The listing builds one solid part. Answer for the finished solid, in the listing's coordinates (mm). A direction names the side the tool comes from. Coordinates: 2 decimals unless noted, no trailing zeros. Write each question's results on one line, items separated by ' | '. Start each with the question number.
(1) Determine the mould class of faces 1 (the face through (168, 590.137, 0)), 2 (the face through (181, 602.837, 5)) for opening direction Z: +Z half, -Z half, draft (parallel to the pull), parting line (faces both ways), or undercut.
(2) A tool of negligible diameter and unlimited length cuts with its end or side. For faces 3 (the face through (168, 477.868, 0)), 4 (the face through (181, 465.168, -5)), 5 (the face through (194, 590.137, 0)), from which of +Z, -Z, +X, -X, +Y, -Y can it reach the whole face along a straight path? Write none if from no direction.
(3) Given pin 1 (3 mm diameter, centred on x = 168.37, z = 0, fed in from -Y); pin 2 (10 mm diameter, centred on x = 175, y = 538.5, fed in from +Z); pin 3 (5 mm diameter, centred on x = 193.77, z = 0, fed in from +Y); pin 4 (3 mm diameter, centred on x = 193.77, z = 0, fed in from +Y), each flat-ended and moving along its own axis, determine where each tip first touches the part or whether it passes through.
(4) Straight lines are drawn through the part: L1, parallel to Y at x = 194, z = -0.25; L2, parallel to Z at x = 203, y = 536; L3, parallel to Z at x = 168.5, y = 570. For each, find the intervals that lie inside material, in ascending order.
```python
from build123d import *

# Parameters (mm, degrees)
BOSS_EXTRUDE1_DEPTH      = 11.1125
BOSS_EXTRUDE1_DEPTH_BACK = 11.1125
SKETCH5_W                = 109.877468776
SKETCH5_H                = 283.051122129
CUT_EXTRUDE2_DEPTH       = 1193.492852366
SKETCH6_W                = 149.121482991
SKETCH6_H                = 108.921761737
CUT_EXTRUDE3_DEPTH       = 1175.662940665
SKETCH7_R                = 4.7625
CUT_EXTRUDE4_DEPTH       = 635
CUT_EXTRUDE5_DEPTH       = 1195.766301895
CUT_EXTRUDE5_DEPTH_BACK  = 1195.766301895
SKETCH8_W                = 149.774750394
SKETCH8_H                = 142.875
SKETCH8_H_2              = 176.125878949
SKETCH9_R                = 1.5875
CUT_EXTRUDE6_DEPTH       = 12.7
CUT_EXTRUDE7_START       = -12.7
SKETCH10_R               = 1.5875
CUT_EXTRUDE7_DEPTH       = 12.7


with BuildPart() as part:
    # Sketch1 → Boss-Extrude1 (new, two sides: drawn at the far end of the back side and taken through both)
    with BuildSketch(Plane.XY.offset(-BOSS_EXTRUDE1_DEPTH_BACK)):
        Polygon((142.42123069, 465.168027231), (219.716026672, 465.168027231), (213.502471629, 1096.967634552), (181.068628681, 1174.337215652), (148.634785732, 1096.967634552), align=None)
    extrude(amount=BOSS_EXTRUDE1_DEPTH + BOSS_EXTRUDE1_DEPTH_BACK)

    # Sketch2 → Cut-Loft1 section 0
    with BuildSketch(Plane.XZ.offset(-465.168027231)):
        with BuildLine():
            Line((142.42123069, 0), (181.068628681, 11.1125))
            Line((181.068628681, 11.1125), (219.716026672, 0))
            Line((219.716026672, 0), (222.70513775, 0))
            Line((222.70513775, 0), (222.70513775, 15.258366339))
            Line((222.70513775, 15.258366339), (137.848628215, 15.258366339))
            Line((137.848628215, 15.258366339), (137.848628215, 0))
            Line((137.848628215, 0), (142.42123069, 0))
        make_face()
    # Sketch3 → Cut-Loft1 section 1
    with BuildSketch(Plane(origin=(0, 1096.967634552, 0), x_dir=(1, 0, 0), z_dir=(0, 1, 0))):
        with BuildLine():
            Line((213.502471629, 0), (181.068628681, -11.1125))
            Line((181.068628681, -11.1125), (148.634785732, 0))
            Line((148.634785732, 0), (137.848628215, 0))
            Line((137.848628215, 0), (137.848628215, -15.258366339))
            Line((137.848628215, -15.258366339), (222.70513775, -15.258366339))
            Line((222.70513775, -15.258366339), (222.70513775, 0))
            Line((222.70513775, 0), (213.502471629, 0))
        make_face()
    cut_loft1 = loft(mode=Mode.SUBTRACT)

    # Mirror1: Cut-Loft1 across plane
    add(cut_loft1.mirror(Plane.XY), mode=Mode.SUBTRACT)

    # Sketch5 → Cut-Extrude2 (cut, through all)
    with BuildSketch(Plane(origin=(-32.103098407, 13.457832356, 93.698704331), x_dir=(0.9470206004067627, 0.045661094409327196, 0.31791043842968925), z_dir=(-0.3211728232668741, 0.1346377834927197, 0.937401026696127))):
        with Locations((219.349244299, 1139.303724701)):
            Rectangle(SKETCH5_W, SKETCH5_H)
    cut_extrude2 = extrude(amount=CUT_EXTRUDE2_DEPTH, mode=Mode.SUBTRACT)

    # Sketch6 → Cut-Extrude3 (cut, through all)
    with BuildSketch(Plane(origin=(69.458274406, 29.117370568, 202.726547902), x_dir=(0.9470206004067623, -0.045661094409327495, -0.31791043842969063), z_dir=(0.3211728232668754, 0.13463778349272, 0.9374010266961263))):
        with Locations((131.752816965, 1118.922251835)):
            Rectangle(SKETCH6_W, SKETCH6_H)
    cut_extrude3 = extrude(amount=CUT_EXTRUDE3_DEPTH, mode=Mode.SUBTRACT)

    # Mirror2: Cut-Extrude2, Cut-Extrude3 across plane
    add(cut_extrude2.mirror(Plane.XY), mode=Mode.SUBTRACT)
    add(cut_extrude3.mirror(Plane.XY), mode=Mode.SUBTRACT)

    # Sketch7 → Cut-Extrude4 (cut)
    with BuildSketch(Plane.XZ.offset(-465.168027231)):
        with Locations(Location((181.068628681, 0, 0), (0, 0, 270))):
            Circle(SKETCH7_R)
    extrude(amount=-CUT_EXTRUDE4_DEPTH, mode=Mode.SUBTRACT)

    # Sketch8 → Cut-Extrude5 (cut, two sides: drawn at the far end of the back side and taken through both)
    with BuildSketch(Plane.XY.offset(-CUT_EXTRUDE5_DEPTH_BACK)):
        with Locations((180.5976389, 674.274715652)):
            Rectangle(SKETCH8_W, SKETCH8_H)
        with Locations((180.5976389, 817.149715652)):
            Rectangle(SKETCH8_W, SKETCH8_H)
        with Locations((180.5976389, 960.024715652)):
            Rectangle(SKETCH8_W, SKETCH8_H)
        with Locations((180.5976389, 1119.525155127)):
            Rectangle(SKETCH8_W, SKETCH8_H_2)
    extrude(amount=CUT_EXTRUDE5_DEPTH + CUT_EXTRUDE5_DEPTH_BACK, mode=Mode.SUBTRACT)

    # Sketch9 → Cut-Extrude6 (cut)
    with BuildSketch(Plane.XZ.offset(-465.168027231)):
        with Locations(Location((168.368628681, 0, 0), (0, 0, 270))):
            Circle(SKETCH9_R)
        with Locations(Location((193.768628681, 0, 0), (0, 0, 270))):
            Circle(SKETCH9_R)
    extrude(amount=-CUT_EXTRUDE6_DEPTH, mode=Mode.SUBTRACT)

    # Sketch10 → Cut-Extrude7 (cut)
    with BuildSketch(Plane(origin=(0, 602.837215652, 0), x_dir=(1, 0, 0), z_dir=(0, 1, 0)).offset(CUT_EXTRUDE7_START)):
        with Locations(Location((168.368628681, 0, 0), (0, 0, 90))):
            Circle(SKETCH10_R)
        with Locations(Location((193.768628681, 0, 0), (0, 0, 90))):
            Circle(SKETCH10_R)
    extrude(amount=CUT_EXTRUDE7_DEPTH, mode=Mode.SUBTRACT)


solid = part.part
```
Established:
1) face 1: undercut | face 2: draft
2) face 3: -Y | face 4: +Z, -Z, +X, -X, -Y | face 5: +Y
3) pin 1: stops at y = 477.87 | pin 2: stops at z = 10.8 | pin 3: stops at y = 602.84 | pin 4: stops at y = 590.14
4) L1: y = 477.87 to 590.14 | L2: z = -4.69 to 4.69 | L3: z = -7.4 to 7.4
